Design review of the part built by this model. Coordinates are the model's own, in mm. A direction names the side the tool comes from. Give positions to 0.01 mm unless a question says otherwise; leave off trailing zeros. Write each loop counter-clockwise with the first axis right and the second up, starting at its lowest first coordinate (ties: lowest second). Pieces come first, ordered by that corner, then holes. Notation, with made-up numbers: (-34.75, 75.5) -> (-18.75, 75.5) arc R14 cw to (-18.75, 85.5) -> close; hole circle Ø10 at (-12, 61). An arc over 180 degrees is marked (long way). Return JSON: item names as keys, results as strings. Group by question number.
from build123d import *

# Parameters (mm, degrees)
SKETCH1_R                = 62.5
SKETCH1_R_2              = 15
BOSS_EXTRUDE1_DEPTH      = 47.5
SKETCH2_R                = 32.5
BOSS_EXTRUDE2_DEPTH      = 50
BOSS_EXTRUDE3_START      = -47.5
BOSS_EXTRUDE3_DEPTH      = 47.5
BOSS_EXTRUDE4_DEPTH      = 100
FILLET1_R                = 25
SKETCH5_W                = 57
SKETCH5_H                = 57
BOSS_EXTRUDE5_DEPTH      = 91
CHAMFER1_SIZE            = 5
SKETCH6_R                = 37.75
CUT_EXTRUDE1_DEPTH       = 100
CUT_EXTRUDE2_DEPTH       = 5
CUT_EXTRUDE2_DEPTH_BACK  = 5
SKETCH8_R                = 45
CUT_EXTRUDE3_DEPTH       = 5
CUT_EXTRUDE3_DEPTH_BACK  = 5
SKETCH9_R                = 45
CUT_EXTRUDE4_DEPTH       = 5
FILLET2_R                = 10
CIRPATTERN1_COUNT        = 4
FILLET2_OF_CIRPATTERN1_R = 10
SKETCH11_R               = 2.35
CUT_EXTRUDE5_DEPTH       = 4
SKETCH12_R               = 1.75
CUT_EXTRUDE6_DEPTH       = 4


with BuildPart() as part:
    # Sketch1 → Boss-Extrude1 (new body)
    with BuildSketch(Plane(origin=(0, 0, 0), x_dir=(0, 0, -1), z_dir=(1, 0, 0))):
        Circle(SKETCH1_R)
        Circle(SKETCH1_R_2, mode=Mode.SUBTRACT)
    extrude(amount=BOSS_EXTRUDE1_DEPTH)

    # Sketch2 → Boss-Extrude2 (add, symmetric)
    with BuildSketch(Plane.XY):
        with BuildLine():
            Line((-35.355339059, 69.644660941), (0, 34.289321881))
            Line((0, 34.289321881), (0, 55))
            ThreePointArc((0, 55), (19.134171618, 151.193976626), (-35.355339059, 69.644660941))
        make_face()
        with Locations((0, 105)):
            Circle(SKETCH2_R, mode=Mode.SUBTRACT)
    extrude(amount=BOSS_EXTRUDE2_DEPTH, both=True)

    # Sketch3 → Boss-Extrude3 (add)
    with BuildSketch(Plane(origin=(47.5, 0, 0), x_dir=(0, 0, -1), z_dir=(1, 0, 0)).offset(BOSS_EXTRUDE3_START)):
        with BuildLine():
            Line((-50, 55), (-50, 62.5))
            Line((-50, 62.5), (50, 62.5))
            Line((50, 62.5), (50, 55))
            Line((50, 55), (50, 37.5))
            ThreePointArc((50, 37.5), (40.792418173, 47.352176503), (29.685855218, 55))
            Line((29.685855218, 55), (-29.685855218, 55))
            ThreePointArc((-29.685855218, 55), (-40.792418173, 47.352176503), (-50, 37.5))
            Line((-50, 37.5), (-50, 55))
        make_face()
    extrude(amount=BOSS_EXTRUDE3_DEPTH)

    # Sketch4 → Boss-Extrude4 (add)
    with BuildSketch(Plane.XY.offset(50)):
        with BuildLine():
            Line((26.339134382, 62.5), (47.5, 62.5))
            Line((47.5, 62.5), (47.5, 89.387505004))
            ThreePointArc((47.5, 89.387505004), (39.291079432, 74.07733716), (26.339134382, 62.5))
        make_face()
    extrude(amount=-BOSS_EXTRUDE4_DEPTH)

    # Fillet1
    fillet1_edges = [part.edges().sort_by_distance(p)[0] for p in [
        (23.75, 37.5, 50),
        (23.75, 37.5, -50),
        (47.5, 89.387505004, 0),
    ]]
    fillet(fillet1_edges, radius=FILLET1_R)

    # Sketch5 → Boss-Extrude5 (add)
    with BuildSketch(Plane.ZY):
        Rectangle(SKETCH5_W, SKETCH5_H)
    extrude(amount=BOSS_EXTRUDE5_DEPTH)

    # Chamfer1
    chamfer1_edges = [part.edges().sort_by_distance(p)[0] for p in [
        (-45.5, -28.5, 28.5),
        (-45.5, 28.5, 28.5),
        (-45.5, 28.5, -28.5),
        (-45.5, -28.5, -28.5),
    ]]
    chamfer(chamfer1_edges, length=CHAMFER1_SIZE)

    # Sketch6 → Cut-Extrude1 (cut)
    with BuildSketch(Plane.XY.offset(50)):
        with Locations((0, 105)):
            Circle(SKETCH6_R)
    extrude(amount=-CUT_EXTRUDE1_DEPTH, mode=Mode.SUBTRACT)

    # Sketch8 → Cut-Extrude2 (cut, two sides: drawn at the far end of the back side and taken through both)
    with BuildSketch(Plane.XY.offset(-CUT_EXTRUDE2_DEPTH_BACK)):
        with Locations((0, 105)):
            Circle(SKETCH8_R)
    extrude(amount=CUT_EXTRUDE2_DEPTH + CUT_EXTRUDE2_DEPTH_BACK, mode=Mode.SUBTRACT)

    # Sketch9 → Cut-Extrude3 (cut, two sides: drawn at the far end of the back side and taken through both)
    with BuildSketch(Plane(origin=(0, 0, -40), x_dir=(-1, 0, 0), z_dir=(0, 0, -1)).offset(-CUT_EXTRUDE3_DEPTH_BACK)):
        with Locations(Location((0, 105, 0), (0, 0, 180))):
            Circle(SKETCH9_R)
    extrude(amount=CUT_EXTRUDE3_DEPTH + CUT_EXTRUDE3_DEPTH_BACK, mode=Mode.SUBTRACT)

    # Sketch10 → Cut-Extrude4 (cut)
    with BuildSketch(Plane.XY.offset(50)):
        with BuildLine():
            Line((-4, 142.399360944), (-4, 145))
            ThreePointArc((-4, 145), (0, 149), (4, 145))
            Line((4, 145), (4, 142.487163458))
            ThreePointArc((4, 142.487163458), (-0.003307195, 142.744592568), (-4, 142.399360944))
        make_face()
    cut_extrude4 = extrude(amount=-CUT_EXTRUDE4_DEPTH, mode=Mode.SUBTRACT)

    # Fillet2
    # the kernel refuses this fillet: 10 mm, written as the material it takes off along each edge
    with BuildSketch(Plane(origin=(-4, 142.537481269, 45), x_dir=(-0.9825908408243521, -0.18578277511139907, 0), z_dir=(0, 0, 1))) as fillet2_piece_1:
        with BuildLine():
            CenterArc((6.893121156, -9.967448048), FILLET2_R, 94.624278966, 49.061773925)
            Line((-1.164720332, -4.045354621), (-1.970504481, -3.453145278))
            ThreePointArc((-1.970504481, -3.453145278), (-1.440084404, -2.233865576), (-0.982590841, 0.185782775))
            Line((-0.982590841, 0.185782775), (0.0806213, 0.996744805))
            ThreePointArc((0.0806213, 0.996744805), (3.043454077, 0.877116383), (6.006286855, 0.996744805))
            Line((6.006286855, 0.996744805), (6.086908155, 0))
        make_face()
    extrude(amount=20.217270387, mode=Mode.SUBTRACT)
    with BuildSketch(Plane(origin=(4, 142.537481269, 45), x_dir=(0.9825908408243521, -0.18578277511139857, 0), z_dir=(0, 0, 1))) as fillet2_piece_2:
        with BuildLine():
            CenterArc((6.893121156, 9.967448048), FILLET2_R, 216.31394711, 49.061773925)
            Line((-1.164720332, 4.045354621), (-1.970504481, 3.453145278))
            ThreePointArc((-1.970504481, 3.453145278), (-1.440084404, 2.233865576), (-0.982590841, -0.185782775))
            Line((-0.982590841, -0.185782775), (0.0806213, -0.996744805))
            ThreePointArc((0.0806213, -0.996744805), (3.043454077, -0.877116383), (6.006286855, -0.996744805))
            Line((6.006286855, -0.996744805), (6.086908155, 0))
        make_face()
    extrude(amount=20.217270387, mode=Mode.SUBTRACT)

    # CirPattern1: Cut-Extrude4 ×4 about axis
    cirpattern1_axis = Axis((0, 105, 0), (0, 0, 1))
    for i in range(1, CIRPATTERN1_COUNT):
        add(cut_extrude4.rotate(cirpattern1_axis, i * 360 / CIRPATTERN1_COUNT), mode=Mode.SUBTRACT)

    # Fillet2 of CirPattern1
    # the kernel refuses this fillet: 10 mm, written as the material it takes off along each edge
    with BuildSketch(Plane(origin=(-37.537481269, 101, 45), x_dir=(0.1857827751113988, -0.9825908408243521, 0), z_dir=(0, 0, 1)), Plane(origin=(4, 67.462518731, 45), x_dir=(0.9825908408243522, 0.18578277511139812, 0), z_dir=(0, 0, 1)), Plane(origin=(37.537481269, 109, 45), x_dir=(-0.1857827751113974, 0.9825908408243524, 0), z_dir=(0, 0, 1))) as fillet2_of_cirpattern1_piece_1:
        with BuildLine():
            CenterArc((6.893121156, -9.967448048), FILLET2_OF_CIRPATTERN1_R, 94.624278966, 49.061773925)
            Line((-1.164720332, -4.045354621), (-1.970504481, -3.453145278))
            ThreePointArc((-1.970504481, -3.453145278), (-1.440084404, -2.233865576), (-0.982590841, 0.185782775))
            Line((-0.982590841, 0.185782775), (0.0806213, 0.996744805))
            ThreePointArc((0.0806213, 0.996744805), (3.043454077, 0.877116383), (6.006286855, 0.996744805))
            Line((6.006286855, 0.996744805), (6.086908155, 0))
        make_face()
    extrude(amount=20.217270387, mode=Mode.SUBTRACT)
    with BuildSketch(Plane(origin=(-37.537481269, 109, 45), x_dir=(0.18578277511140218, 0.9825908408243516, 0), z_dir=(0, 0, 1)), Plane(origin=(-4, 67.462518731, 45), x_dir=(-0.982590840824351, 0.1857827751114053, 0), z_dir=(0, 0, 1)), Plane(origin=(37.537481269, 101, 45), x_dir=(-0.18578277511140162, -0.9825908408243517, 0), z_dir=(0, 0, 1))) as fillet2_of_cirpattern1_piece_2:
        with BuildLine():
            CenterArc((6.893121156, 9.967448048), FILLET2_OF_CIRPATTERN1_R, 216.31394711, 49.061773925)
            Line((-1.164720332, 4.045354621), (-1.970504481, 3.453145278))
            ThreePointArc((-1.970504481, 3.453145278), (-1.440084404, 2.233865576), (-0.982590841, -0.185782775))
            Line((-0.982590841, -0.185782775), (0.0806213, -0.996744805))
            ThreePointArc((0.0806213, -0.996744805), (3.043454077, -0.877116383), (6.006286855, -0.996744805))
            Line((6.006286855, -0.996744805), (6.086908155, 0))
        make_face()
    extrude(amount=20.217270387, mode=Mode.SUBTRACT)

    # Sketch11 → Cut-Extrude5 (cut)
    with BuildSketch(Plane.XY.offset(45)):
        with Locations((0, 145.621023241)):
            Circle(SKETCH11_R)
        with Locations((40.621023241, 105)):
            Circle(SKETCH11_R)
        with Locations((0, 64.378976759)):
            Circle(SKETCH11_R)
        with Locations((-40.621023241, 105)):
            Circle(SKETCH11_R)
    extrude(amount=-CUT_EXTRUDE5_DEPTH, mode=Mode.SUBTRACT)

    # Sketch12 → Cut-Extrude6 (cut)
    with BuildSketch(Plane.XY.offset(41)):
        with Locations((0, 145.621023241)):
            Circle(SKETCH12_R)
        with Locations((40.621023241, 105)):
            Circle(SKETCH12_R)
        with Locations((0, 64.378976759)):
            Circle(SKETCH12_R)
        with Locations((-40.621023241, 105)):
            Circle(SKETCH12_R)
    extrude(amount=-CUT_EXTRUDE6_DEPTH, mode=Mode.SUBTRACT)


solid = part.part
Q1. Take a section at A-A, the plane z = 0. Give the boundary of the cut face in (x, y).
Q2. Insertion check: pin 1 (4 mm diameter, centred on x = -40.62, y = 105, fed in from -Z); pin 2 (1 mm diameter, centred on x = -13.5, z = -3.5, fed in from +Y); pin 3 (12 mm diameter, centred on x = 11, z = 38.5, fed in from -Y). Each pin has a flat end and moves straight along its axis. Give the tip position at first contact, or say it passes through.
Q3. Take a section at C-C, the plane x = -63.5. Give the boundary of the cut face in (y, z).
Q4. Tool access review of faces 4 (the face through (-45, 0, -28.5)), 5 (the face through (20.765, 65.077, -0.07)), 6 (the face through (6.17, 143.413, 47.465)): name each direction out of +Z, -Z, +X, -X, +Y, -Y from which nothing blocks a thin tool from reaching the whole face with its end or side.
Q5. Mouldability with a two-part tool opening along Z and no side actions: class faces 1 (the face through (-10, 142, 5)), 2 (the face through (41, 107, 41)), 3 (the face through (-17.925, 52.214, 0.7)) as +Z half, -Z half, draft (parallel to the pull), parting line (faces both ways), or undercut.
Q6. Take a section at B-B, the plane x = -29.5. Count the separate pieces of the cut face and the enclosed holes in it, plus the area to 3 significant figures.
Q7. Take a section at D-D, the plane y = 47.5. Give the boundary of the cut face in (x, z).
Q8. For L1, parallel to X at y = -45, z = -25.5; L2, parallel to Y at x = -34, z = 47; L3, parallel to X at y = 126, z = -48, list the stretches that pass through material, from the lowest coordinate up. Write a range as from..to.
Final values:
{
 "1": {"outline": "(-91, -28.5) -> (0, -28.5) -> (0, -62.5) -> (47.5, -62.5) -> (47.5, -15) -> (0, -15) -> (0, 15) -> (47.5, 15) -> (47.5, 85.8) arc R25 cw to (48.33, 92.2) arc R50 ccw (long way) to (-35.36, 69.64) -> (0, 34.29) -> (0, 28.5) -> (-91, 28.5) -> close; hole circle Ø90 at (0, 105)"},
 "2": {"pin 1": "stops at z = -50", "pin 2": "stops at y = 153.28", "pin 3": "stops at y = -53.39"},
 "3": {"outline": "(-28.5, -23.5) -> (-23.5, -28.5) -> (23.5, -28.5) -> (28.5, -23.5) -> (28.5, 23.5) -> (23.5, 28.5) -> (-23.5, 28.5) -> (-28.5, 23.5) -> close"},
 "4": {"face 4": "-Z, -X, -Y", "face 5": "none", "face 6": "+Z"},
 "5": {"face 1": "undercut", "face 2": "+Z half", "face 3": "draft"},
 "6": {"separate pieces": "3", "enclosed holes": "0", "area": "6,230 mm²"},
 "7": {"outline": "(-13.21, -50) -> (47.5, -50) -> (47.5, 50) -> (-13.21, 50) -> close"},
 "8": {"L1": "x = 0..47.5", "L2": "y = 68.29..88.6, 121.4..141.66", "L3": "x = -45.38..-31.37, 31.37..45.38"}
}
